```python
from build123d import *

# Parameters (mm, degrees)
SKETCH_1_W             = 50
SKETCH_1_H             = 30
EXTRUDE_1_DEPTH        = 15
SKETCH_2_W             = 18
SKETCH_2_H             = 10.25
CUT_EXTRUDE_1_DEPTH    = 5
SKETCH_3_W             = 30
SKETCH_3_H             = 26
CUT_EXTRUDE_2_DEPTH    = 13
SKETCH_4_W             = 7.5
SKETCH_4_H             = 13
CUT_EXTRUDE_3_DEPTH    = 50
SKETCH_5_W             = 7.5
SKETCH_5_H             = 13
CUT_EXTRUDE_4_DEPTH    = 50
CUT_EXTRUDE_5_DEPTH    = 50
SKETCH_7_R             = 1.25
CUT_EXTRUDE_6_DEPTH    = 50
PATTERN_LINEAR_1_COUNT = 2
PATTERN_LINEAR_1_PITCH = 45
SKETCH_8_R             = 1
CUT_EXTRUDE_7_DEPTH    = 5
PATTERN_LINEAR_2_COUNT = 2
PATTERN_LINEAR_2_PITCH = 25


with BuildPart() as part:
    # Эскиз1 → Бобышка-Вытянуть1 (new body)
    with BuildSketch(Plane.XY):
        Rectangle(SKETCH_1_W, SKETCH_1_H)
    extrude(amount=EXTRUDE_1_DEPTH)

    # Эскиз2 → Вырез-Вытянуть1 (cut)
    with BuildSketch(Plane(origin=(0, 15, 0), x_dir=(1, 0, 0), z_dir=(0, 1, 0))):
        with Locations((0, -9.875)):
            Rectangle(SKETCH_2_W, SKETCH_2_H)
    extrude(amount=-CUT_EXTRUDE_1_DEPTH, mode=Mode.SUBTRACT)

    # Эскиз3 → Вырез-Вытянуть2 (cut)
    with BuildSketch(Plane.XY.offset(15)):
        Rectangle(SKETCH_3_W, SKETCH_3_H)
    extrude(amount=-CUT_EXTRUDE_2_DEPTH, mode=Mode.SUBTRACT)

    # Эскиз4 → Вырез-Вытянуть3 (cut)
    with BuildSketch(Plane(origin=(0, 15, 0), x_dir=(1, 0, 0), z_dir=(0, 1, 0))):
        with Locations((-21.25, -6.5)):
            Rectangle(SKETCH_4_W, SKETCH_4_H)
    extrude(amount=-CUT_EXTRUDE_3_DEPTH, mode=Mode.SUBTRACT)

    # Эскиз5 → Вырез-Вытянуть4 (cut)
    with BuildSketch(Plane(origin=(0, 15, 0), x_dir=(1, 0, 0), z_dir=(0, 1, 0))):
        with Locations((21.25, -6.5)):
            Rectangle(SKETCH_5_W, SKETCH_5_H)
    extrude(amount=-CUT_EXTRUDE_4_DEPTH, mode=Mode.SUBTRACT)

    # Эскиз6 → Вырез-Вытянуть5 (cut)
    with BuildSketch(Plane.XZ.offset(15)):
        with BuildLine():
            Line((-5, 15), (5, 15))
            ThreePointArc((5, 15), (0, 10), (-5, 15))
        make_face()
    extrude(amount=-CUT_EXTRUDE_5_DEPTH, mode=Mode.SUBTRACT)

    # Эскиз7 → Вырез-Вытянуть6 (cut)
    with BuildSketch(Plane.XY.offset(15)):
        with Locations((22.5, 0)):
            Circle(SKETCH_7_R)
    cut_extrude_6 = extrude(amount=-CUT_EXTRUDE_6_DEPTH, mode=Mode.SUBTRACT)

    # Линейный массив1: Вырез-Вытянуть6 ×2
    with Locations(*[(-i * PATTERN_LINEAR_1_PITCH, 0, 0) for i in range(1, PATTERN_LINEAR_1_COUNT)]):
        add(cut_extrude_6, mode=Mode.SUBTRACT)

    # Эскиз8 → Вырез-Вытянуть7 (cut)
    with BuildSketch(Plane(origin=(0, 15, 0), x_dir=(1, 0, 0), z_dir=(0, 1, 0))):
        with Locations(Location((-12.5, -8.7, 0), (0, 0, 270))):
            Circle(SKETCH_8_R)
    cut_extrude_7 = extrude(amount=-CUT_EXTRUDE_7_DEPTH, mode=Mode.SUBTRACT)

    # Линейный массив2: Вырез-Вытянуть7 ×2
    with Locations(*[(i * PATTERN_LINEAR_2_PITCH, 0, 0) for i in range(1, PATTERN_LINEAR_2_COUNT)]):
        add(cut_extrude_7, mode=Mode.SUBTRACT)


solid = part.part
```
Verification items for the finished model (mm, model axes). A direction names the side the tool comes from. Give positions to 0.01 mm unless a question says otherwise; leave off trailing zeros. Write each loop counter-clockwise with the first axis right and the second up, starting at its lowest first coordinate (ties: lowest second). Pieces come first, ordered by that corner, then holes. Notation, with made-up numbers: (-12.75, 40) - (43.25, 40) arc R16 ccw to (43.25, 61) - close; hole circle Ø5 at (-23.5, -5.5). An arc over 180 degrees is marked (long way). Put each result on its own line as item: value.
Q1. Set-up check for faces 1 (the face through (0, 0, 2)), 2 (the face through (12.117, 14.014, 9.624)), 3 (the face through (0, 14, 4.75)): record each of +Z, -Z, +X, -X, +Y, -Y from which the full face is reachable in a straight line by a thin tool's end or side.
Result:
face 1: +Z
face 2: +Y
face 3: +Z, +Y
Q2. Section check C-C on z = 13.5. Record the cut outline in (x, y), and give its area (3 significant figures).
Result:
outline: (-25, -15) - (-4.77, -15) - (-4.77, -13) - (-15, -13) - (-15, 13) - (-9, 13) - (-9, 15) - (-25, 15) - close; (4.77, -15) - (25, -15) - (25, 15) - (9, 15) - (9, 13) - (15, 13) - (15, -13) - (4.77, -13) - close; hole circle Ø2.5 at (-22.5, 0); hole circle Ø2.5 at (22.5, 0)
area: 655 mm2
Q3. Section check D-D on x = 0. Record the cut outline in (y, z), and give its area (3 significant figures).
Result:
outline: (-15, 0) - (15, 0) - (15, 4.75) - (13, 4.75) - (13, 2) - (-13, 2) - (-13, 10) - (-15, 10) - close
area: 81.5 mm2
Q4. Mould release check, pull along X, two halves, no side actions. Record for faces 4 (the face through (-25, 0, 14)), 5 (the face through (-9, 14, 10)), 6 (the face through (21, 0, 13)): released by +X, released by -X, zero draft, split by the parting line, or undercut.
Result:
face 4: released by -X
face 5: undercut
face 6: zero draft
Q5. Scan lines: probe 1 along X at (y, z) = (14.15, 8.7); probe 2 along Y at (x, z) = (22.5, 14.3); probe 3 along X at (y, z) = (5.5, 11.5). Record each from-to range of solid material in increasing order. Write a range as from..to.
Result:
probe 1: -17.5..-13.5, -11.5..-9, 9..11.5, 13.5..17.5
probe 2: -15..-1.25, 1.25..15
probe 3: -17.5..-15, 15..17.5
Q6. Depth check by flat-ended pin: P1, Ø2, axis at y = 14.5, z = 10.5, coming from the -X side; P2, Ø1, axis at x = 4, y = 14.5, coming from the +Z side; P3, Ø4, axis at x = 21, y = 5.5, coming from the -Z side. Enter the tip coordinate at first touch or a pass-through.
Result:
P1: x = -17.5
P2: z = 4.75
P3: z = 13
Q7. Section check A-A on z = 3.5. Record the cut outline in (x, y), and give its area (3 significant figures).
Result:
outline: (-17.5, -15) - (17.5, -15) - (17.5, 15) - (-17.5, 15) - close; hole (-15, -13) - (15, -13) - (15, 13) - (-15, 13) - close
area: 270 mm2
Q8. Section check B-B on x = -12.5. Record the cut outline in (y, z), and give its area (3 significant figures).
Result:
outline: (-15, 0) - (15, 0) - (15, 7.7) - (13, 7.7) - (13, 2) - (-13, 2) - (-13, 15) - (-15, 15) - close; (13, 9.7) - (15, 9.7) - (15, 15) - (13, 15) - close
area: 108 mm2
